Can you work these out from the model? Positions are in its coordinate system, mm. A direction names the side the tool comes from. Coordinates: 2 decimals unless noted, no trailing zeros. Loops run counter-clockwise (first coordinate to the right, second up) from the corner with the lowest first, then second, coordinate; pieces in that order, holes last. Notation, with made-up numbers: (-39, 78) -> (2, 78) arc R25 ccw to (2, 96) -> close; hole circle Ø1 at (-19.5, 89). An arc over 180 degrees is marked (long way). Put each result on its own line as item: value. Start each with the question number.
Item 1: If we section it at A-A on y = -116.5: Please give me the cut outline in (x, z).
Item 2: If we section it at C-C on z = 274.5: Please give me the cut outline in (x, y), plus the area to 3 significant figures.
Item 3: Please list where these lines run through material, in increasing order: L1, parallel to Z at x = -153, y = -262; L2, parallel to Y at x = -160, z = -266; L3, parallel to X at y = -186.5, z = -84.5. Write a range as from..to.
Item 4: We'd pull the mould along Z, two halves only. Please class faces 4 (the flat face through (-152, -12, 360)), 5 (the flat face through (-101, -275, -350)), 6 (the flat face through (-152, -148, -80)): pulls with the +Z half, pulls with the -Z half, needs draft (parallel to the pull), parting line crosses it, or undercut.
Item 5: Will these pins go through, and if not, where does the flat tip stop? P1, Ø1, axis at x = -124.5, y = -180, coming from the +Z side; P2, Ø8, axis at x = -169.5, z = -213.5, coming from the -Y side; P3, Ø8, axis at x = -168, z = 44, coming from the +Y side.
Item 6: If we section it at D-D on y = -210: Please give me the cut outline in (x, z), plus the area to 3 significant figures.
Item 7: For faces 1 (the flat face through (-152, -148, -340)), 2 (the flat face through (-152, -148, 180)), 3 (the flat face through (-152, -136, -360)), which set-ups out of +Z, -Z, +X, -X, +Y, -Y let a thin tool reach every point of the face, with its end or its side?
Item 8: If we section it at B-B on x = -87.5: Please give me the cut outline in (y, z).
```python
from build123d import *

# Parameters (mm, degrees)
F0_W     = 300
F0_H     = 720
F1_DEPTH = 25
F2_W     = 300
F2_H     = 20
F3_DEPTH = 250
F4_R     = 100
F5_W     = 300
F5_H     = 20
F6_DEPTH = 250
F7_R     = 100


with BuildPart() as f1:
    # F0 (on Front) → F1 (new body)
    with BuildSketch(Plane.XZ):
        with Locations((-150, 0)):
            Rectangle(F0_W, F0_H)
    extrude(amount=F1_DEPTH)

    # F2 (on face) → F3 (join)
    with BuildSketch(Plane.XZ.offset(25)):
        with Locations((-150, -350)):
            Rectangle(F2_W, F2_H)
    extrude(amount=F3_DEPTH)

    # F4
    f4_edges = [f1.edges().sort_by_distance(p)[0] for p in [
        (-300, -275, -350),
    ]]
    fillet(f4_edges, radius=F4_R)

    # F5 (on face) → F6 (join)
    with BuildSketch(Plane.XZ.offset(25)):
        with Locations((-150, -90)):
            Rectangle(F5_W, F5_H)
        with Locations((-150, 170)):
            Rectangle(F5_W, F5_H)
    extrude(amount=F6_DEPTH)

    # F7
    f7_edges = [f1.edges().sort_by_distance(p)[0] for p in [
        (-300, -275, 170),
        (-300, -275, -90),
    ]]
    fillet(f7_edges, radius=F7_R)


solid = f1.part
```
Solutions:
1. outline: (-300, -360) -> (0, -360) -> (0, -340) -> (-300, -340) -> close; (-300, -100) -> (0, -100) -> (0, -80) -> (-300, -80) -> close; (-300, 160) -> (0, 160) -> (0, 180) -> (-300, 180) -> close
2. outline: (-300, -25) -> (0, -25) -> (0, 0) -> (-300, 0) -> close
2. area: 7,500 mm^2
3. L1: -360..-340, -100..-80, 160..180
3. L2: -25..0
3. L3: -299.34..0
4. face 4: pulls with the +Z half
4. face 5: needs draft
4. face 6: undercut
5. P1: z = 180
5. P2: y = -25
5. P3: y = 0
6. outline: (-293.67, -360) -> (0, -360) -> (0, -340) -> (-293.67, -340) -> close; (-293.67, -100) -> (0, -100) -> (0, -80) -> (-293.67, -80) -> close; (-293.67, 160) -> (0, 160) -> (0, 180) -> (-293.67, 180) -> close
6. area: 17,600 mm^2
7. face 1: +X, -X, -Y
7. face 2: +Z, +X, -X, -Y
7. face 3: -Z, +X, -X, +Y, -Y
8. outline: (-275, -360) -> (0, -360) -> (0, 360) -> (-25, 360) -> (-25, 180) -> (-275, 180) -> (-275, 160) -> (-25, 160) -> (-25, -80) -> (-275, -80) -> (-275, -100) -> (-25, -100) -> (-25, -340) -> (-275, -340) -> close
